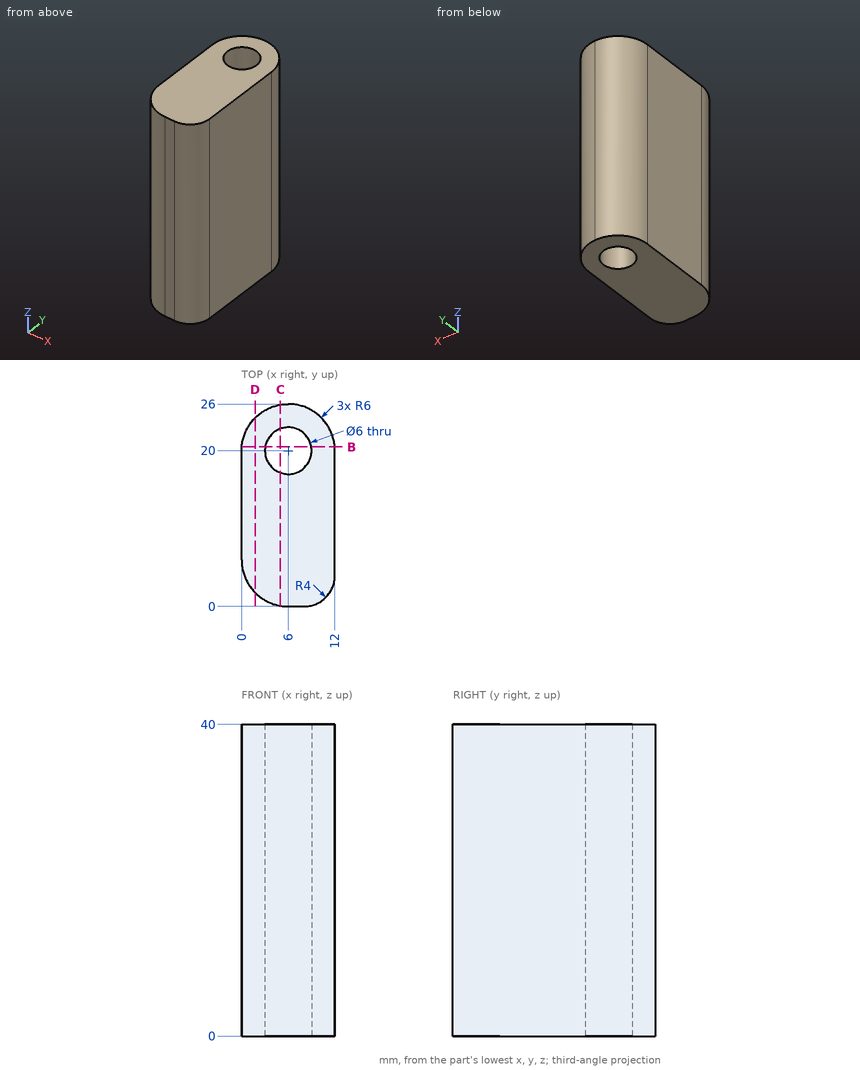
For this review, use the dimensioned drawing (mm, ordinates from the lowest corner) and the shaded views. Coordinates: 2 decimals unless noted, no trailing zeros. Write each loop counter-clockwise with the first axis right and the second up, starting at its lowest first coordinate (ties: lowest second). Pieces come first, ordered by that corner, then holes. Notation, with made-up numbers: (63, -13) -> (80, -13) arc R18 ccw to (80, 1) -> close; hole circle Ø2 at (41, 45.25). An arc over 180 degrees is marked (long way). Write each question's results on one line, items separated by ' | '. Start each with the question number.
(1) Take a section at D-D on x = 1.75. Write out the cut boundary in (y, z).
(2) Take a section at C-C on x = 5. Write out the cut boundary in (y, z), and give its area (3 significant figures).
(3) Clearance check with flat-ended pins moving along their axes: P1, Ø4, axis at y = 10.5, z = 11.5, coming from the -X side; P2, Ø1, axis at x = 2, z = 4.5, coming from the +Y side. State where each tip first meets the part, or that it passes through.
(4) For line 1 along Y through (x, z) = (6, 12.5); line 2 along X through (y, z) = (20.25, 19.5) (1 decimal); line 3 along Y through (x, z) = (7.25, 9), list the stretches that pass through material, from the lowest coordinate up. Write a range as from..to.
(5) Take a section at B-B on y = 20.5. Write out the cut boundary in (x, z).
Results found:
1) outline: (1.76, 0) -> (24.24, 0) -> (24.24, 40) -> (1.76, 40) -> close
2) outline: (0.08, 0) -> (17.17, 0) -> (17.17, 40) -> (0.08, 40) -> close; (22.83, 0) -> (25.92, 0) -> (25.92, 40) -> (22.83, 40) -> close | area: 807 mm2
3) P1: stops at x = 0 | P2: stops at y = 24.87
4) line 1: y = 0..17, 23..26 | line 2: x = 0..3, 9..12 | line 3: y = 0..17.27, 22.73..25.87
5) outline: (0.02, 0) -> (3.04, 0) -> (3.04, 40) -> (0.02, 40) -> close; (8.96, 0) -> (11.98, 0) -> (11.98, 40) -> (8.96, 40) -> close
